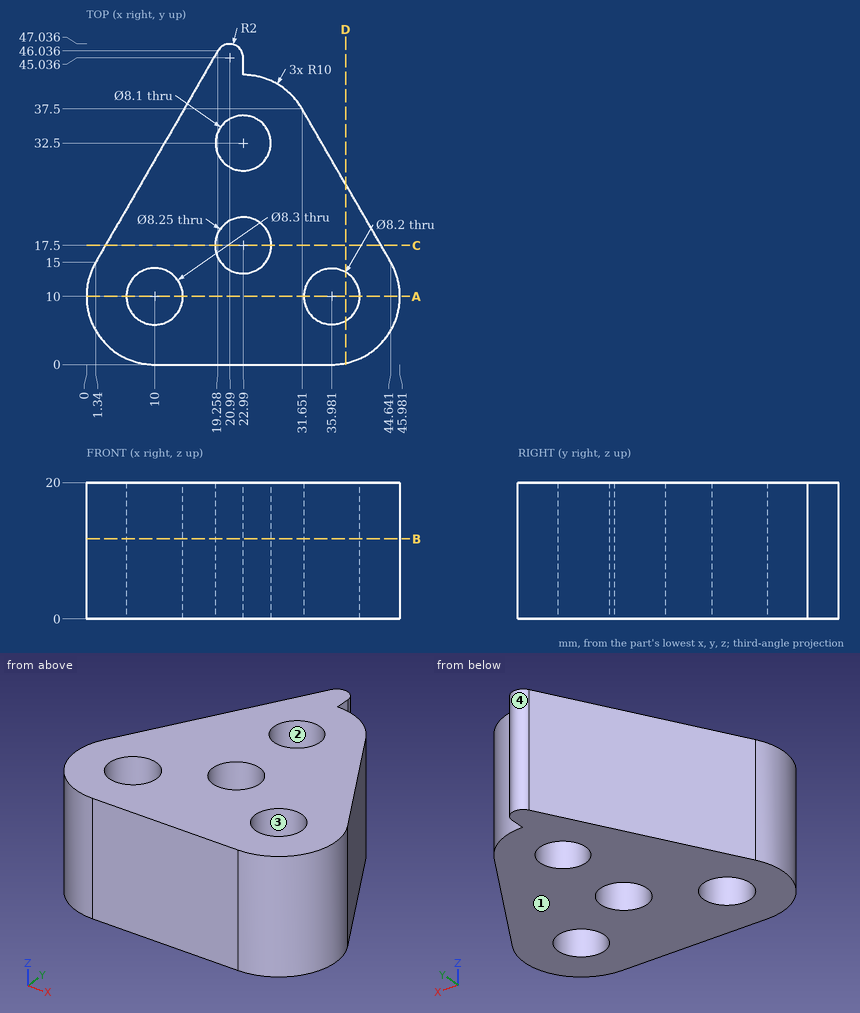
The figure shows three views and two pictorial views of one solid part (mm, origin at its lowest corner). Answer the questions. Coordinates: 2 decimals unless noted, no trailing zeros. Loops run counter-clockwise (first coordinate to the right, second up) from the corner with the lowest first, then second, coordinate; pieces in that order, holes last. Notation, with made-up numbers: M 67,84 L 80,84 A8 ccw 80,92 Z; hole C 9.5,13.25 d8. An arc over 180 degrees is marked long. Use CSV: the item, a comma, the result in double quotes. Start each with the question number.
(1) Find section C-C, the plane y = 17.5. Give the vertices of the cut face in (x, z) (1 decimal), then the cut area to 3 significant figures.
(2) For a pull along X with two mould halves and no side action, classify the marked faces 1, 2, 3 and 4 as +X half, -X half, draft (parallel to the pull), parting line (faces both ways), or undercut.
(3) Find section A-A, the plane y = 10. Give the vertices of the cut face in (x, z).
(4) Consider line 1 (X direction, y = 7, z = 11) (1 decimal); line 2 (Y direction, x = 26.5, z = 16) (1 decimal); line 3 (X direction, y = 12.5, z = 5.5) (1 decimal). Determine where each line is inside the solid, lowest interval first.
(5) Find section B-B, the plane z = 11.75. State how many separate pieces and enclosed holes the cut face has, then the cut area to 3 significant figures.
(6) Find section D-D, the plane x = 38. Give the vertices of the cut face in (y, z), then the cut area to 3 significant figures.
(7) Given pin 1 Ø4 at (x, z) = (17.5, 17) entering from +Y; pin 2 Ø12 at (y, z) = (29, 12) entering from +X; pin 3 Ø2 at (y, z) = (14.5, 10.5) entering from -X, each flat-ended and moving along its own axis, determine where each tip first touches the part or whether it passes through.
Recorded:
1,outline,"M 2.8,0 L 18.9,0 L 18.9,20 L 2.8,20 Z; M 27.1,0 L 43.2,0 L 43.2,20 L 27.1,20 Z"
1,area,"643 mm^2"
2,face 1,"draft"
2,face 2,"undercut"
2,face 3,"undercut"
2,face 4,"parting line"
3,outline,"M 0,0 L 5.85,0 L 5.85,20 L 0,20 Z; M 14.15,0 L 31.88,0 L 31.88,20 L 14.15,20 Z; M 40.08,0 L 45.98,0 L 45.98,20 L 40.08,20 Z"
4,line 1,"x = 0.5 to 7.1, 12.9 to 33.2, 38.8 to 45.5"
4,line 2,"y = 0 to 15.3, 19.7 to 30.5, 34.5 to 41.9"
4,line 3,"x = 0.3 to 6.7, 13.3 to 32.7, 39.2 to 45.7"
5,separate pieces,"1"
5,enclosed holes,"4"
5,area,"1,200 mm^2"
6,outline,"M 0.21,0 L 6.43,0 L 6.43,20 L 0.21,20 Z; M 13.57,0 L 26.5,0 L 26.5,20 L 13.57,20 Z"
6,area,"383 mm^2"
7,pin 1,"stops at y = 46.37"
7,pin 2,"stops at x = 40.02"
7,pin 3,"stops at x = 0.63"
